```python
from build123d import *

# Parameters (mm, degrees)
F2_DEPTH = 1.875
F4_W     = 7
F4_H     = 4.75
F5_DEPTH = 25


with BuildPart() as f2:
    # F1 (on Top) → F2 (new body, symmetric)
    with BuildSketch(Plane.XY):
        Polygon((-25, -25), (0, -25), (0, 0), (-3.5, 0), (-3.5, 5.8333333333), (-1.875, 5.8333333333), (-1.875, 9.5833333333), (-3.5, 9.5833333333), (-3.5, 15.4166666667), (-1.875, 15.4166666667), (-1.875, 19.1666666667), (-3.5, 19.1666666667), (-3.5, 25), (-25, 25), align=None)
    extrude(amount=F2_DEPTH, both=True)

    # F3: F2 across face


with BuildPart() as f2_1:
    add(f2.part)
    add(f2.part.mirror(Plane(origin=(0, -12.5, 0), x_dir=(0, 1, 0), z_dir=(1, 0, 0))))

    # F4 (on face) → F5 (cut)
    with BuildSketch(Plane.XY.offset(1.875)):
        with Locations((0, -7.5416666667)):
            Rectangle(F4_W, F4_H)
        with Locations((0, -17.4583333333)):
            Rectangle(F4_W, F4_H)
    extrude(amount=-F5_DEPTH, mode=Mode.SUBTRACT)


solid = f2_1.part
```
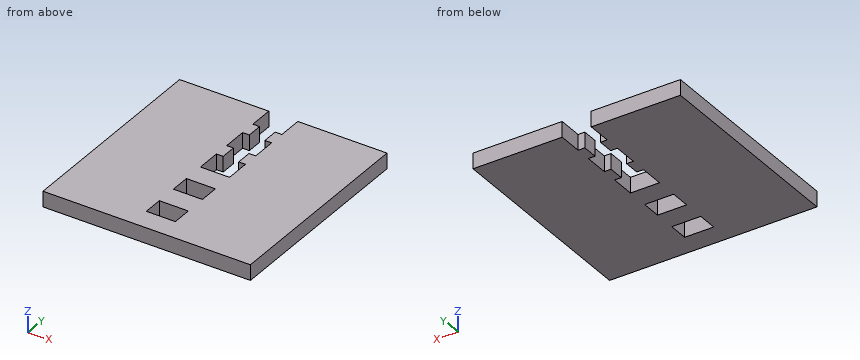
Model file for the job. Use its own axes, mm. Coordinates: 2 decimals unless noted, no trailing zeros. Order: outer loops, then holes, each group sorted by start corner. A loop starts at its lowest first (then second) coordinate and runs counter-clockwise, first axis right, second up. Notation, with made-up numbers: (-19.5, 19) -> (10.5, 19) arc R8 ccw to (10.5, 33) -> close; hole circle Ø1 at (-16, 14.25). An arc over 180 degrees is marked (long way). Answer as a JSON object with one key per item and string values. Group by question number.
1) Cut at A-A, the plane y = 18.5. Write the cut outline in (x, z) (3 decimals), then the cut area to 3 significant figures.
2) Flat gauge pins, fed straight in: pin 1 (0.8 mm diameter, centred on x = -2.5, z = 0.5, fed in from +Y); pin 2 (1.9 mm diameter, centred on x = 0, z = 0, fed in from +Y). Where does each tip first touch, or does it go through?
3) Cut at B-B, the plane z = -0.55. Count the separate pieces of the cut face and the enclosed holes in it, then the cut area to 3 significant figures.
4) Drill centre lines: L1, parallel to Y at x = 0.5, z = -1.15; L2, parallel to X at y = 23, z = -0.7; L3, parallel to X at y = 6.5, z = 0.7 (3 decimals). Where is each one in solid material? Low to high.
Check values:
{
 "1": {"outline": "(-25, -1.875) -> (-1.875, -1.875) -> (-1.875, 1.875) -> (-25, 1.875) -> close; (1.875, -1.875) -> (25, -1.875) -> (25, 1.875) -> (1.875, 1.875) -> close", "area": "173 mm²"},
 "2": {"pin 1": "stops at y = 19.17", "pin 2": "stops at y = 0"},
 "3": {"separate pieces": "1", "enclosed holes": "2", "area": "2,280 mm²"},
 "4": {"L1": "y = -25 to -19.83, -15.08 to -9.92, -5.17 to 0", "L2": "x = -25 to -3.5, 3.5 to 25", "L3": "x = -25 to -1.875, 1.875 to 25"}
}
